Verification items for the finished model (mm, model axes). A direction names the side the tool comes from. Round coordinates to 2 decimals unless told otherwise and drop trailing zeros. Write each loop counter-clockwise with the first axis right and the second up, starting at its lowest first coordinate (ties: lowest second). Pieces come first, ordered by that corner, then holes. Notation, with made-up numbers: M 40,7 L 59,7 A18 cw 59,31 Z; hole C -29,83.25 d5. An arc over 180 degrees is marked long. One line per item, written item: value. Start each with the question number.
Item 1: Section check A-A, the plane z = -13.84. Record the cut outline in (x, y).
Item 2: Draft check along Z on faces 5 (the face through (-9.643, 7.465, 7.801)), 6 (the face through (-24, 5, -21.5)), 7 (the face through (3, 8, -16)). Enter one of: +Z half, -Z half, draft (parallel to the pull), parting line (faces both ways), or undercut.
Item 3: Tool access check on faces 1 (the face through (12.5, 7, 19)), 2 (the face through (9.763, 7.465, -7.801)), 3 (the face through (-2.88, 8, 16)), 4 (the face through (-8, 3, -20.45)). Record the directions out of +Z, -Z, +X, -X, +Y, -Y that give a thin tool (end or side, any length) a straight path to the whole face; none if there is none.
Item 4: Section check D-D, the plane z = 18.5. Record the cut outline in (x, y), then the cut area to 3 significant figures.
Item 5: Section check B-B, the plane y = 6.25. Record the cut outline in (x, z), then the cut area to 3 significant figures.
Item 6: Section check C-C, the plane x = 27.34. Record the cut outline in (y, z), then the cut area to 3 significant figures.
Item 7: Gauge pin test, flat ends, axial feed: pin 1 (6 mm diameter, centred on x = 16, z = -9, fed in from -Y); pin 2 (6 mm diameter, centred on x = 2.5, y = 5.5, fed in from -Z); pin 3 (5.5 mm diameter, centred on x = 8, y = 2.5, fed in from +Z). Record the tip position at first contact, or that the pin passes through.
Item 8: Thickness scan on probe 1 along X at (y, z) = (6.75, -13.84); probe 2 along X at (y, z) = (4, -13.84); probe 3 along X at (y, z) = (8.25, 13). Record the ranges inside material, lowest first. Write a range as from..to.
from build123d import *

# Parameters (mm, degrees)
SKETCH_1_W           = 70
SKETCH_1_H           = 43
EXTRUDE_1_DEPTH      = 10
SKETCH_4_R           = 2.5
CUT_EXTRUDE_1_DEPTH  = 10
SKETCH_5_R           = 2.5
CUT_EXTRUDE_2_DEPTH  = 10
SKETCH_8_W           = 24.88
SKETCH_8_H           = 5
CUT_EXTRUDE_4_DEPTH  = 57.338264084
SKETCH_11_R          = 20.45
SKETCH_11_R_2        = 12.45
EXTRUDE_1_2_DEPTH    = 5
CUT_EXTRUDE_6_DEPTH  = 5
CUT_EXTRUDE_7_DEPTH  = 5
SKETCH_16_W          = 5.88
SKETCH_16_H          = 11
CUT_EXTRUDE_8_DEPTH  = 5
SKETCH_17_W          = 5.88
SKETCH_17_H          = 8.352111755
CUT_EXTRUDE_9_DEPTH  = 5
CUT_EXTRUDE_10_DEPTH = 5
CUT_EXTRUDE_11_DEPTH = 5


with BuildPart() as part:
    # 草圖1 → Extrude 1 (new body)
    with BuildSketch(Plane(origin=(0, 0, 0), x_dir=(1, 0, 0), z_dir=(0, 1, 0))):
        Rectangle(SKETCH_1_W, SKETCH_1_H)
    extrude(amount=EXTRUDE_1_DEPTH)

    # 草圖4 → 除料-伸長1 (cut)
    with BuildSketch(Plane(origin=(0, 10, 0), x_dir=(1, 0, 0), z_dir=(0, 1, 0))):
        with Locations(Location((-27.34, 13.84, 0), (0, 0, 270))):
            Circle(SKETCH_4_R)
    extrude(amount=-CUT_EXTRUDE_1_DEPTH, mode=Mode.SUBTRACT)

    # 草圖5 → 除料-伸長2 (cut)
    with BuildSketch(Plane(origin=(0, 10, 0), x_dir=(1, 0, 0), z_dir=(0, 1, 0))):
        with Locations(Location((27.34, 13.84, 0), (0, 0, 270))):
            Circle(SKETCH_5_R)
    extrude(amount=-CUT_EXTRUDE_2_DEPTH, mode=Mode.SUBTRACT)

    # 草圖8 → 除料-伸長4 (cut, through all)
    with BuildSketch(Plane.XY.offset(21.5)):
        with Locations((0.06, 7.5)):
            Rectangle(SKETCH_8_W, SKETCH_8_H)
    extrude(amount=-CUT_EXTRUDE_4_DEPTH, mode=Mode.SUBTRACT)

    # 草圖11 → Extrude 1 2 (add)
    with BuildSketch(Plane(origin=(0, 5, 0), x_dir=(1, 0, 0), z_dir=(0, 1, 0))):
        with Locations((0.06, 0)):
            Circle(SKETCH_11_R)
        with Locations((0.06, 0)):
            Circle(SKETCH_11_R_2, mode=Mode.SUBTRACT)
    extrude(amount=EXTRUDE_1_2_DEPTH)

    # 草圖14 → 除料-伸長6 (cut)
    with BuildSketch(Plane(origin=(0, 5, 0), x_dir=(1, 0, 0), z_dir=(0, 1, 0))):
        Polygon((0.06, -20.45), (12.5, -20.45), (12.5, -21.5), (-12.38, -21.5), (-12.38, -20.45), align=None)
    extrude(amount=-CUT_EXTRUDE_6_DEPTH, mode=Mode.SUBTRACT)

    # 草圖15 → 除料-伸長7 (cut)
    with BuildSketch(Plane(origin=(0, 5, 0), x_dir=(1, 0, 0), z_dir=(0, 1, 0))):
        Polygon((0.06, 20.45), (12.5, 20.45), (12.5, 21.5), (-12.38, 21.5), (-12.38, 20.45), align=None)
    extrude(amount=-CUT_EXTRUDE_7_DEPTH, mode=Mode.SUBTRACT)

    # 草圖16 → 除料-伸長8 (cut)
    with BuildSketch(Plane(origin=(0, 10, 0), x_dir=(1, 0, 0), z_dir=(0, 1, 0))):
        with Locations((0.06, 17.597888245)):
            Rectangle(SKETCH_16_W, SKETCH_16_H)
    extrude(amount=-CUT_EXTRUDE_8_DEPTH, mode=Mode.SUBTRACT)

    # 草圖17 → 除料-伸長9 (cut)
    with BuildSketch(Plane(origin=(0, 10, 0), x_dir=(1, 0, 0), z_dir=(0, 1, 0))):
        with Locations((0.06, -16.273944123)):
            Rectangle(SKETCH_17_W, SKETCH_17_H)
    extrude(amount=-CUT_EXTRUDE_9_DEPTH, mode=Mode.SUBTRACT)

    # 草圖19 → 除料-伸長10 (cut)
    with BuildSketch(Plane(origin=(0, 5, 0), x_dir=(1, 0, 0), z_dir=(0, 1, 0))):
        Polygon((-2.88, 20.237561612), (-2.88, 20.45), (2.98755849, 20.45), (3, 20.237561612), align=None)
    extrude(amount=-CUT_EXTRUDE_10_DEPTH, mode=Mode.SUBTRACT)

    # 草圖20 → 除料-伸長11 (cut)
    with BuildSketch(Plane(origin=(0, 5, 0), x_dir=(1, 0, 0), z_dir=(0, 1, 0))):
        Polygon((3, -20.237561612), (3, -20.45), (-2.887827835, -20.45), (-2.88, -20.237561612), align=None)
    extrude(amount=-CUT_EXTRUDE_11_DEPTH, mode=Mode.SUBTRACT)


solid = part.part
Response values:
1. outline: M -35,0 L -29.84,0 L -29.84,10 L -35,10 Z; M -24.84,0 L 24.84,0 L 24.84,10 L 3,10 L 3,5 L -2.88,5 L -2.88,10 L -24.84,10 Z; M 29.84,0 L 35,0 L 35,10 L 29.84,10 Z
2. face 5: undercut
2. face 6: -Z half
2. face 7: draft
3. face 1: +Z, +Y
3. face 2: +Y
3. face 3: +Z, -Z, +Y
3. face 4: -Z, +Y, -Y
4. outline: M -35,0 L 35,0 L 35,10 L 12.5,10 L 12.5,5 L 8.78,5 L 8.78,10 L 3,10 L 3,5 L -2.88,5 L -2.88,10 L -8.66,10 L -8.66,5 L -12.38,5 L -12.38,10 L -35,10 Z
4. area: 633 mm2
5. outline: M -35,-21.5 L -12.38,-21.5 L -12.38,-16.23 A20.45 ccw -2.88,-20.24 L -2.88,-12.1 A12.45 cw -12.38,-0.5 L -12.38,0.5 A12.45 cw -2.88,12.1 L -2.88,20.24 A20.45 ccw -12.38,16.23 L -12.38,21.5 L -35,21.5 Z; M 3,-20.24 A20.45 ccw 12.5,-16.23 L 12.5,-21.5 L 35,-21.5 L 35,21.5 L 12.5,21.5 L 12.5,16.23 A20.45 ccw 3,20.24 L 3,12.1 A12.45 cw 12.5,0.5 L 12.5,-0.5 A12.45 cw 3,-12.1 Z; hole C -27.34,-13.84 d5; hole C 27.34,-13.84 d5
5. area: 2,270 mm2
6. outline: M 0,-21.5 L 10,-21.5 L 10,-16.34 L 0,-16.34 Z; M 0,-11.34 L 10,-11.34 L 10,21.5 L 0,21.5 Z
6. area: 380 mm2
7. pin 1: stops at y = 0
7. pin 2: stops at z = -20.45
7. pin 3: stops at z = 20.45
8. probe 1: x = -35..-29.84, -24.84..-2.88, 3..24.84, 29.84..35
8. probe 2: x = -35..-29.84, -24.84..24.84, 29.84..35
8. probe 3: x = -35..-2.88, 3..35
